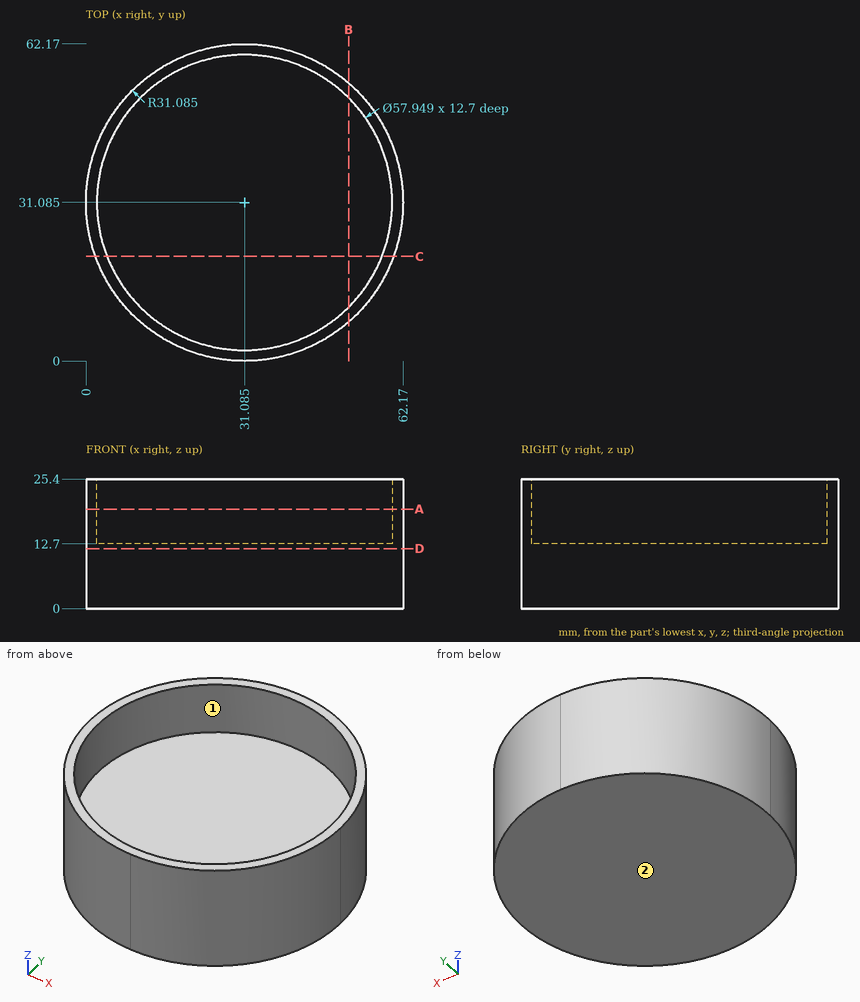
Geometry check sheet. Reference: drawing and pictorial views, mm from the part's lowest x, y, z. Coordinates: 2 decimals unless noted, no trailing zeros. Write each loop counter-clockwise with the first axis right and the second up, starting at its lowest first coordinate (ties: lowest second). Pieces come first, ordered by that corner, then holes. Notation, with made-up numbers: M 42,64 L 62,64 A18 cw 62,90 Z; hole C 31,50 d4. An arc over 180 degrees is marked long. One line per question, with ' | ' between items.
1) Release check for a two-part mould opening along Y. For the marked faces 1 and 2 record: +Y half, -Y half, draft (parallel to the pull), parting line (faces both ways), or undercut.
Solutions:
face 1: undercut | face 2: draft
2) Sectioned sample at B-B on x = 51.5. Record the cut outline in (y, z).
Solutions:
outline: M 7.64,0 L 54.53,0 L 54.53,25.4 L 51.65,25.4 L 51.65,12.7 L 10.52,12.7 L 10.52,25.4 L 7.64,25.4 Z
3) Sectioned sample at D-D on z = 11.75. Record the cut outline in (x, y) (1 decimal).
Solutions:
outline: M 0,31.1 A31.1 ccw 31.1,0 A31.1 ccw 62.2,31.1 A31.1 ccw 31.1,62.2 A31.1 ccw Z
4) Sectioned sample at C-C on y = 20.5. Record the cut outline in (x, z).
Solutions:
outline: M 1.86,0 L 60.31,0 L 60.31,25.4 L 58.06,25.4 L 58.06,12.7 L 4.11,12.7 L 4.11,25.4 L 1.86,25.4 Z
5) Material ranges on L1, parallel to X at y = 23.5, z = 13.5; L2, parallel to Z at x = 50, y = 44.5; L3, parallel to Y at x = 51.5, z = 18.5 (1 decimal), recorded low to high.
Solutions:
L1: 0.94 to 3.12, 59.05 to 61.23 | L2: 0 to 12.7 | L3: 7.6 to 10.5, 51.6 to 54.5
6) Sectioned sample at A-A on z = 19.5. Record the cut outline in (x, y) (1 decimal).
Solutions:
outline: M 0,31.1 A31.1 ccw 31.1,0 A31.1 ccw 62.2,31.1 A31.1 ccw 31.1,62.2 A31.1 ccw Z; hole C 31.1,31.1 d57.9
7) Depth check by flat-ended pin: pin 1 Ø5 at (y, z) = (54, 9) entering from -X; pin 2 Ø10 at (x, z) = (24, 3.5) entering from +Y; pin 3 Ø1.5 at (y, z) = (20, 10) entering from -X. Enter the tip coordinate at first touch or a pass-through.
Solutions:
pin 1: x = 7.64 | pin 2: y = 62.1 | pin 3: x = 1.77
